Autodesk Inventor part; units mm, degrees
ref_plane "Work Plane1" through (13.5, 0, 0) normal (1, 0, 0) x (0, 0, -1)
ref_plane "YZ Plane" through (0, 0, 0) normal (1, 0, 0) x (0, 1, 0)
ref_plane "XZ Plane" through (0, 0, 0) normal (0, 1, 0) x (-1, 0, 0)
sketch "Sketch1" plane through (0, 0, 0) normal (1, 0, 0) x (0, 1, 0)
  circle A0 centre (0, 0) radius 1.75
  dimension "d0" = 3.5
extrude "Extrusion1" add sketch "Sketch1" along normal blind 10
sketch "Sketch2" plane through (10, 0, 0) normal (1, 0, 0) x (0, 0, -1)
  circle A0 centre (0, 0) radius 2.625
  dimension "d3" = 5.25
extrude "Extrusion2" add sketch "Sketch2" along normal blind 3.5
ref_plane "Work Plane1" through (13.5, 0, 0) normal (1, 0, 0) x (0, 0, -1)
sketch "Sketch3" plane through (13.5, 0, 0) normal (1, 0, 0) x (0, 0, -1)
  line L0 (0, -1.4) -> (-1.2124, -0.7)
  line L1 (-1.2124, -0.7) -> (-1.2124, 0.7)
  line L2 (-1.2124, 0.7) -> (0, 1.4)
  line L3 (0, 1.4) -> (1.2124, 0.7)
  line L4 (1.2124, 0.7) -> (1.2124, -0.7)
  line L5 (1.2124, -0.7) -> (0, -1.4)
  point P0 (0, 0)
  point P1 (0, 0)
  dimension "d9" = 2.8
  dimension "d10" = 1.2124
extrude "Extrusion3" cut sketch "Sketch3" against normal blind 1.75
fillet "Fillet2" radius 0.2 1 edges at (13.5, 0, 2.625)
properties part number "M3.5" material "Iron, Cast"
The listing builds one solid part. Answer for the finished solid, in the listing's coordinates (mm). A direction names the side the tool comes from. Give positions to 0.01 mm unless a question says otherwise; leave off trailing zeros. Loops run counter-clockwise (first coordinate to the right, second up) from the corner with the lowest first, then second, coordinate; pieces in that order, holes last.
Item 1: A cutting plane is placed at A-A (y = 0). Give the vertices of the cut face in (x, z) (3 decimals).
Derived:
outline: (0, -1.75) - (10, -1.75) - (10, -2.625) - (13.3, -2.625) arc R0.2 ccw to (13.5, -2.425) - (13.5, -1.212) - (11.75, -1.212) - (11.75, 1.212) - (13.5, 1.212) - (13.5, 2.425) arc R0.2 ccw to (13.3, 2.625) - (10, 2.625) - (10, 1.75) - (0, 1.75) - close
Item 2: A cutting plane is placed at B-B (x = 2.75). Give the vertices of the cut face in (y, z).
Derived:
outline: circle Ø3.5 at (0, 0)
Item 3: Each of these flat-tipped pins is pushed along its axis until it touches: pin 1 Ø0.7 at (y, z) = (0, 0) entering from +X; pin 2 Ø1 at (x, z) = (4, 0.5) entering from +Y; pin 3 Ø3 at (y, z) = (-1.5, -1) entering from -X. Where does it stop, or does it pass through?
Derived:
pin 1: stops at x = 11.75
pin 2: stops at y = 1.75
pin 3: stops at x = 0
Item 4: Find the intervals of material crossed by line 1 along Z through (x, y) = (12, 0.1); line 2 along X through (y, z) = (-0.9, -0.1); line 3 along X through (y, z) = (1.45, 1.55), in increasing order.
Derived:
line 1: z = -2.62 to -1.21, 1.21 to 2.62
line 2: x = 0 to 11.75
line 3: x = 10 to 13.5
Item 5: Determine the mould class of faces 1 (the flat face through (12.64, -1.05, -0.61)), 2 (the cylindrical face through (11.6, -0.8, -2.5)), 3 (the flat face through (10, -2, -1)) for opening direction Y: +Y half, -Y half, draft (parallel to the pull), parting line (faces both ways), or undercut.
Derived:
face 1: undercut
face 2: parting line
face 3: draft
Item 6: A tool of negligible diameter and unlimited length cuts with its end or side. For faces 4 (the cylindrical face through (4.93, 1.617, 0.67)), 5 (the flat face through (13.5, 1, -1)), 6 (the flat face through (13, 0, 1.212)), from which of +Z, -Z, +X, -X, +Y, -Y can it reach the whole face along a straight path? Write none if from no direction.
Derived:
face 4: -X
face 5: +Z, -Z, +X, +Y, -Y
face 6: +X
